Design review of the part built by this model. Coordinates are the model's own, in mm. A direction names the side the tool comes from. Coordinates: 2 decimals unless noted, no trailing zeros. Loops run counter-clockwise (first coordinate to the right, second up) from the corner with the lowest first, then second, coordinate; pieces in that order, holes last. Notation, with made-up numbers: (66.25, 81.25) -> (92.25, 81.25) arc R20 cw to (92.25, 97.25) -> close; hole circle Ø5 at (81.5, 55.5). An arc over 180 degrees is marked (long way). Answer in a Markdown table with one row per item.
```python
from build123d import *

# Parameters (mm, degrees)
ESBO_O2_W                = 51
ESBO_O2_H                = 50
RESSALTO_EXTRUS_O2_DEPTH = 6
CORTE_EXTRUS_O1_DEPTH    = 25
CORTE_EXTRUS_O3_DEPTH    = 25
ESBO_O5_R                = 1.5
RESSALTO_EXTRUS_O3_DEPTH = 6
ESBO_O8_R                = 1.5
CORTE_EXTRUS_O6_DEPTH    = 37.211186117
CHANFRO2_SIZE            = 1.5


with BuildPart() as part:
    # Esboço2 → Ressalto-extrusão2 (new body)
    with BuildSketch(Plane(origin=(0, 0, 0), x_dir=(1, 0, 0), z_dir=(0, 1, 0))):
        Rectangle(ESBO_O2_W, ESBO_O2_H)
    extrude(amount=RESSALTO_EXTRUS_O2_DEPTH)

    # Esboço3 → Corte-extrusão1 (cut)
    with BuildSketch(Plane.XY.offset(25)):
        Polygon((-25.5, 0.6), (25.5, 5.06192184), (25.5, 6), (-25.5, 6), align=None)
    extrude(amount=-CORTE_EXTRUS_O1_DEPTH, mode=Mode.SUBTRACT)

    # Esboço4 → Corte-extrusão3 (cut)
    with BuildSketch(Plane(origin=(0, 0, -25), x_dir=(-1, 0, 0), z_dir=(0, 0, -1))):
        Polygon((-25.5, 0.6), (25.5, 5.06192184), (25.5, 6), (-25.5, 6), align=None)
    extrude(amount=-CORTE_EXTRUS_O3_DEPTH, mode=Mode.SUBTRACT)

    # Esboço5 → Ressalto-extrusão3 (add)
    with BuildSketch(Plane.XZ):
        with Locations(Location((0, 6, 0), (0, 0, 270))):
            Circle(ESBO_O5_R)
        with Locations(Location((0, 15, 0), (0, 0, 270))):
            Circle(ESBO_O5_R)
        with Locations(Location((0, -15, 0), (0, 0, 270))):
            Circle(ESBO_O5_R)
        with Locations(Location((0, -6, 0), (0, 0, 270))):
            Circle(ESBO_O5_R)
    extrude(amount=-RESSALTO_EXTRUS_O3_DEPTH)

    # Esboço8 → Corte-extrusão6 (cut, through all)
    with BuildSketch(Plane.XZ):
        with Locations(Location((20, 20, 0), (0, 0, 270))):
            Circle(ESBO_O8_R)
        with Locations(Location((-20, -20, 0), (0, 0, 270))):
            Circle(ESBO_O8_R)
    extrude(amount=-CORTE_EXTRUS_O6_DEPTH, mode=Mode.SUBTRACT)

    # Chanfro2
    chanfro2_edges = [part.edges().sort_by_distance(p)[0] for p in [
        (20, 0, 21.5),
        (-20, 0, -18.5),
    ]]
    chamfer(chanfro2_edges, length=CHANFRO2_SIZE)


solid = part.part
```
(1) Tool access review of faces 1 (the flat face through (0, 6, 6)), 2 (the cylindrical face through (1.487, 4.313, -14.805)): name each direction out of +Z, -Z, +X, -X, +Y, -Y from which nothing blocks a thin tool from reaching the whole face with its end or side.
Evaluation:
| item | result |
|---|---|
| face 1 | +Z, -Z, +X, -X, +Y |
| face 2 | +Y |
(2) Take a section at A-A on x = 20. Give the boundary of the cut face in (y, z).
Evaluation:
| item | result |
|---|---|
| outline | (0, -25) -> (1.08, -25) -> (1.08, 0) -> (4.58, 0) -> (4.58, 18.5) -> (1.5, 18.5) -> (0, 17) -> close; (0, 23) -> (1.5, 21.5) -> (4.58, 21.5) -> (4.58, 25) -> (0, 25) -> close |
(3) To check wall thickness, follow probe 1 along Z at (x, y) = (-20, 3.9); probe 2 along Y at (x, z) = (-19, -16); probe 3 along Z at (x, y) = (-10.5, 2.1). State the ranges of each line that lie inside material, in increasing order.
Evaluation:
| item | result |
|---|---|
| probe 1 | z = -25 to -21.5, -18.5 to 0 |
| probe 2 | y = 0 to 4.49 |
| probe 3 | z = -25 to 0 |
(4) Draft analysis for pull direction Z (two halves, no side actions). For faces 3 (the cylindrical face through (1.487, 4.313, -5.805)), 4 (the flat face through (0, 0, 0)), 5 (the flat face through (5, 2, 25)), state which applies: pulls with the +Z half, pulls with the -Z half, needs draft (parallel to the pull), parting line crosses it, or undercut.
Evaluation:
| item | result |
|---|---|
| face 3 | undercut |
| face 4 | needs draft |
| face 5 | pulls with the +Z half |
(5) Take a section at D-D on x = -8. Give the boundary of the cut face in (y, z), and give its area (3 significant figures).
Evaluation:
| item | result |
|---|---|
| outline | (0, -25) -> (3.53, -25) -> (3.53, 0) -> (2.13, 0) -> (2.13, 25) -> (0, 25) -> close |
| area | 142 mm² |
(6) Take a section at C-C on z = 6.5. Give the boundary of the cut face in (x, y), and give its area (3 significant figures).
Evaluation:
| item | result |
|---|---|
| outline | (-25.5, 0) -> (25.5, 0) -> (25.5, 5.06) -> (1.41, 2.95) -> (1.41, 6) -> (-1.41, 6) -> (-1.41, 2.71) -> (-25.5, 0.6) -> close |
| area | 153 mm² |
(7) For pin 1 (1.5 mm diameter, centred on x = 19, z = -3, fed in from +Y); pin 2 (3.5 mm diameter, centred on x = -20, z = -20, fed in from +Y); pin 3 (8 mm diameter, centred on x = -11, z = 3, fed in from +Y), all flat-tipped, find the tip position at first contact; note any pin that passes through.
Evaluation:
| item | result |
|---|---|
| pin 1 | stops at y = 1.23 |
| pin 2 | stops at y = 4.73 |
| pin 3 | stops at y = 4.02 |
(8) Take a section at B-B on z = -20. Give the boundary of the cut face in (x, y), and give its area (3 significant figures).
Evaluation:
| item | result |
|---|---|
| outline | (-25.5, 0) -> (-23, 0) -> (-21.5, 1.5) -> (-21.5, 4.71) -> (-25.5, 5.06) -> close; (-18.5, 1.5) -> (-17, 0) -> (25.5, 0) -> (25.5, 0.6) -> (-18.5, 4.45) -> close |
| area | 128 mm² |
